CAD build for the part. Positions are in the model's coordinates, mm. A direction names the side the tool comes from. Round coordinates to 2 decimals unless told otherwise and drop trailing zeros. Loops run counter-clockwise (first coordinate to the right, second up) from the corner with the lowest first, then second, coordinate; pieces in that order, holes last.
```python
from build123d import *

# Parameters (mm, degrees)
SKETCH1_W           = 155.4
SKETCH1_H           = 86.98
SKETCH1_W_2         = 152.4
SKETCH1_H_2         = 83.98
SKETCH1_W_3         = 146
SKETCH1_H_3         = 77.58
BOSS_EXTRUDE1_DEPTH = 1.5
SKETCH1_3_W         = 155.4
SKETCH1_3_H         = 86.98
SKETCH1_3_W_2       = 152.4
SKETCH1_3_H_2       = 83.98
BOSS_EXTRUDE2_DEPTH = 15
FILLET1_R           = 2
FILLET2_R           = 1
BOSS_EXTRUDE3_DEPTH = 1.5
BOSS_EXTRUDE4_START = 83.98
SKETCH2_3_R         = 2.675
BOSS_EXTRUDE4_DEPTH = 0.85


with BuildPart() as part:
    # Sketch1 → Boss-Extrude1 (new body)
    with BuildSketch(Plane.XY.offset(120.134907759)):
        with Locations((-26.721041987, -25.88696544)):
            Rectangle(SKETCH1_W, SKETCH1_H)
        with Locations((-26.721041987, -25.88696544)):
            Rectangle(SKETCH1_W_2, SKETCH1_H_2, mode=Mode.SUBTRACT)
        with Locations((-26.721041987, -25.88696544)):
            Rectangle(SKETCH1_W_2, SKETCH1_H_2)
        with Locations((-26.721041987, -25.88696544)):
            Rectangle(SKETCH1_W_3, SKETCH1_H_3, mode=Mode.SUBTRACT)
    extrude(amount=BOSS_EXTRUDE1_DEPTH)

    # Sketch1<3> → Boss-Extrude2 (add)
    with BuildSketch(Plane.XY.offset(120.134907759)):
        with Locations((-26.721041987, -25.88696544)):
            Rectangle(SKETCH1_3_W, SKETCH1_3_H)
        with Locations((-26.721041987, -25.88696544)):
            Rectangle(SKETCH1_3_W_2, SKETCH1_3_H_2, mode=Mode.SUBTRACT)
    extrude(amount=-BOSS_EXTRUDE2_DEPTH)

    # Fillet1
    fillet1_edges = [part.edges().sort_by_distance(p)[0] for p in [
        (50.978958013, -69.37696544, 113.384907759),
        (-104.421041987, -69.37696544, 113.384907759),
        (-104.421041987, 17.60303456, 113.384907759),
        (50.978958013, 17.60303456, 113.384907759),
    ]]
    fillet(fillet1_edges, radius=FILLET1_R)

    # Fillet2
    fillet2_edges = [part.edges().sort_by_distance(p)[0] for p in [
        (-26.721041987, -64.67696544, 121.634907759),
        (-99.721041987, -25.88696544, 121.634907759),
        (-26.721041987, 12.90303456, 121.634907759),
        (46.278958013, -25.88696544, 121.634907759),
        (-26.721041987, -69.37696544, 105.134907759),
        (-26.721041987, -69.37696544, 121.634907759),
        (50.978958013, -25.88696544, 105.134907759),
        (-104.421041987, -25.88696544, 105.134907759),
        (-26.721041987, 17.60303456, 105.134907759),
        (50.393171575, -68.791179003, 105.134907759),
        (50.393171575, 17.017248122, 105.134907759),
        (-103.835255549, 17.017248122, 105.134907759),
        (-103.835255549, -68.791179003, 105.134907759),
        (-104.421041987, -25.88696544, 121.634907759),
        (50.978958013, -25.88696544, 121.634907759),
        (-26.721041987, 17.60303456, 121.634907759),
        (50.393171575, -68.791179003, 121.634907759),
        (50.393171575, 17.017248122, 121.634907759),
        (-103.835255549, 17.017248122, 121.634907759),
        (-103.835255549, -68.791179003, 121.634907759),
    ]]
    fillet(fillet2_edges, radius=FILLET2_R)

    # Sketch2 → Boss-Extrude3 (add)
    with BuildSketch(Plane(origin=(0, -67.87696544, 0), x_dir=(1, 0, 0), z_dir=(0, 1, 0))):
        with BuildLine():
            Line((-96.971041987, -110.65805506), (-93.471041987, -110.65805506))
            ThreePointArc((-93.471041987, -110.65805506), (-92.788258088, -109.747197065), (-92.546041987, -108.634907759))
            ThreePointArc((-92.546041987, -108.634907759), (-96.333331293, -106.20212386), (-96.971041987, -110.65805506))
        make_face()
        with BuildLine():
            Line((40.028958013, -110.65805506), (43.528958013, -110.65805506))
            ThreePointArc((43.528958013, -110.65805506), (44.211741912, -109.747197065), (44.453958013, -108.634907759))
            ThreePointArc((44.453958013, -108.634907759), (40.666668707, -106.20212386), (40.028958013, -110.65805506))
        make_face()
    extrude(amount=BOSS_EXTRUDE3_DEPTH)

    # Sketch2<3> → Boss-Extrude4 (add)
    with BuildSketch(Plane(origin=(0, -67.87696544, 0), x_dir=(1, 0, 0), z_dir=(0, 1, 0)).offset(BOSS_EXTRUDE4_START)):
        with BuildLine():
            Line((-96.971041987, -110.65805506), (-93.471041987, -110.65805506))
            ThreePointArc((-93.471041987, -110.65805506), (-92.788258088, -109.747197065), (-92.546041987, -108.634907759))
            ThreePointArc((-92.546041987, -108.634907759), (-96.333331293, -106.20212386), (-96.971041987, -110.65805506))
        make_face()
        with Locations((41.778958013, -108.634907759)):
            Circle(SKETCH2_3_R)
    extrude(amount=-BOSS_EXTRUDE4_DEPTH)


solid = part.part
```
Item 1: 3-axis set-ups, long thin cutter, end or side, ignore diameter. For faces 1 (the flat face through (-28, 17.603, 113)), 2 (the cylindrical face through (43.01, 15.68, 111.01)), 3 (the flat face through (-102.921, -26, 113)): which of +Z, -Z, +X, -X, +Y, -Y reach the whole face in a straight line?
Answers follow:
face 1: +Z, -Z, +X, -X, +Y
face 2: none
face 3: -Z
Item 2: Cut at A-A, the plane x = 34.5. Give the cut face in (y, z), plus the area to 3 significant figures.
Answers follow:
outline: (-69.38, 106.13) arc R1 ccw to (-68.38, 105.13) - (-67.88, 105.13) - (-67.88, 120.13) - (-64.68, 120.13) - (-64.68, 120.63) arc R1 ccw to (-65.68, 121.63) - (-68.38, 121.63) arc R1 ccw to (-69.38, 120.63) - close; (12.9, 120.13) - (16.1, 120.13) - (16.1, 105.13) - (16.6, 105.13) arc R1 ccw to (17.6, 106.13) - (17.6, 120.63) arc R1 ccw to (16.6, 121.63) - (13.9, 121.63) arc R1 ccw to (12.9, 120.63) - close
area: 57.8 mm2
Item 3: Two-plate mould, pull along Y, no slides. Class faces 4 (the flat face through (-95, 15.253, 108)), 5 (the flat face through (-28, -67.877, 113)), 6 (the flat face through (-104.421, -26, 113)), 7 (the flat face through (-28, -69.377, 113)): released by +Y, released by -Y, zero draft, split by the parting line, or undercut.
Answers follow:
face 4: undercut
face 5: undercut
face 6: zero draft
face 7: released by -Y
Item 4: Probe line 1 (X direction, y = 4, z = 112.25); line 2 (Y direction, x = -25, z = 115.25); line 3 (X direction, y = -8.5, z = 120.75). List the from-to ranges inside material, lowest first.
Answers follow:
line 1: x = -104.42 to -102.92, 49.48 to 50.98
line 2: y = -69.38 to -67.88, 16.1 to 17.6
line 3: x = -104.41 to -99.73, 46.29 to 50.97
Item 5: Cut at B-B, the plane z = 118.25. Give the cut face in (x, y).
Answers follow:
outline: (-104.42, -67.38) arc R2 ccw to (-102.42, -69.38) - (48.98, -69.38) arc R2 ccw to (50.98, -67.38) - (50.98, 15.6) arc R2 ccw to (48.98, 17.6) - (-102.42, 17.6) arc R2 ccw to (-104.42, 15.6) - close; hole (-102.92, -67.88) - (49.48, -67.88) - (49.48, 16.1) - (-102.92, 16.1) - close
Item 6: Cut at C-C, the plane y = -8. Give the cut face in (x, z).
Answers follow:
outline: (-104.42, 106.13) arc R1 ccw to (-103.42, 105.13) - (-102.92, 105.13) - (-102.92, 120.13) - (-99.72, 120.13) - (-99.72, 120.63) arc R1 ccw to (-100.72, 121.63) - (-103.42, 121.63) arc R1 ccw to (-104.42, 120.63) - close; (46.28, 120.13) - (49.48, 120.13) - (49.48, 105.13) - (49.98, 105.13) arc R1 ccw to (50.98, 106.13) - (50.98, 120.63) arc R1 ccw to (49.98, 121.63) - (47.28, 121.63) arc R1 ccw to (46.28, 120.63) - close
